Read the model definition and answer for the solid it produces. Units are mm, in the model's axes. Face numbers are marked on the shaded views. A direction names the side the tool comes from. Round coordinates to 2 decimals unless told otherwise and drop trailing zeros. Loops run counter-clockwise (first coordinate to the right, second up) from the corner with the lowest first, then second, coordinate; pieces in that order, holes last. Notation, with made-up numbers: (32, -3.5) - (80, -3.5) arc R16 cw to (80, 22.5) - close; hole circle Ø4 at (74, -4.75). An arc over 180 degrees is marked (long way). Use CSV: the item, a comma, the result in double quotes. Start each with the question number.
1. Determine the mould class of the marked faces 1, 2, 3 and 4 for opening direction Y: +Y half, -Y half, draft (parallel to the pull), parting line (faces both ways), or undercut.
2. Consider line 1 along X through (y, z) = (35.5, 0.85); line 2 along X through (y, z) = (1, 2.8); line 3 along Y through (x, z) = (10, 0.8). Determine where each line is inside the solid, lowest interval first.
3. Given pin 1 Ø1.5 at (y, z) = (42, 1) entering from +X; pin 2 Ø1.5 at (y, z) = (37, 1.5) entering from -X; pin 3 Ø1 at (y, z) = (28, 0.5) entering from -X, each flat-ended and moving along its own axis, determine where each tip first touches the part or whether it passes through.
4. Find section B-B (x = 9.75). Give the vertices of the cut face in (y, z), and give its area (3 significant figures).
5. Find section A-A (z = 1.5). Give the vertices of the cut face in (x, y).
6. A tool of negligible diameter and unlimited length cuts with its end or side. For the marked faces 5 and 6, from which of +Z, -Z, +X, -X, +Y, -Y can it reach the whole face along a straight path? Write none if from no direction.
7. Find section C-C (y = 14). Give the vertices of the cut face in (x, z).
from build123d import *

# Parameters (mm, degrees)
PAD_DEPTH    = 3
SKETCH001_R  = 1.5
PAD001_DEPTH = 6


with BuildPart() as part:
    # Sketch → Pad (new body)
    with BuildSketch(Plane.XY):
        Polygon((-9.25, -33), (14.25, -33), (14.25, -11.5), (7, -11.5), (7, 33), (4, 33), (4, 43), (-4, 43), (-4, 33), (-7, 33), (-7, -11.5), (-9.25, -11.5), align=None)
    extrude(amount=PAD_DEPTH)

    # Sketch001 → Pad001 (join, symmetric)
    with BuildSketch(Plane.YZ):
        with Locations((40, 1.5)):
            Circle(SKETCH001_R)
    extrude(amount=PAD001_DEPTH, both=True)


solid = part.part
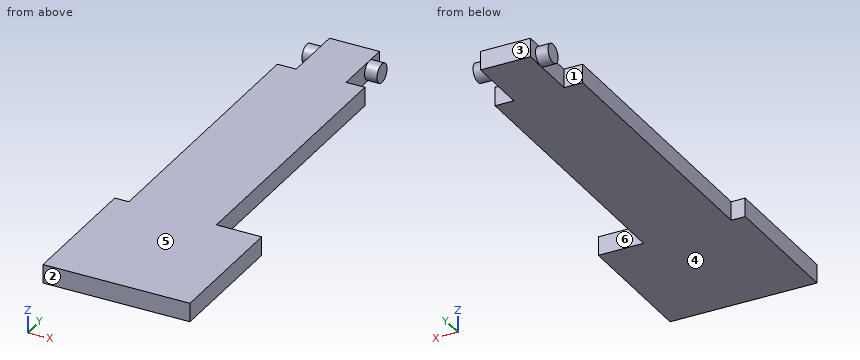
Filled sheet:
1,face 1,"undercut"
1,face 2,"-Y half"
1,face 3,"+Y half"
1,face 4,"draft"
2,line 1,"x = -4 to 4"
2,line 2,"x = -7 to 7"
2,line 3,"y = -33 to -11.5"
3,pin 1,"stops at x = 6"
3,pin 2,"stops at x = -4"
3,pin 3,"stops at x = -7"
4,outline,"(-33, 0) - (-11.5, 0) - (-11.5, 3) - (-33, 3) - close"
4,area,"64.5 mm²"
5,outline,"(-9.25, -33) - (14.25, -33) - (14.25, -11.5) - (7, -11.5) - (7, 33) - (4, 33) - (4, 38.5) - (6, 38.5) - (6, 41.5) - (4, 41.5) - (4, 43) - (-4, 43) - (-4, 41.5) - (-6, 41.5) - (-6, 38.5) - (-4, 38.5) - (-4, 33) - (-7, 33) - (-7, -11.5) - (-9.25, -11.5) - close"
6,face 5,"+Z, +X, -X, +Y, -Y"
6,face 6,"+Z, -Z, +X, +Y"
7,outline,"(-7, 0) - (7, 0) - (7, 3) - (-7, 3) - close"
